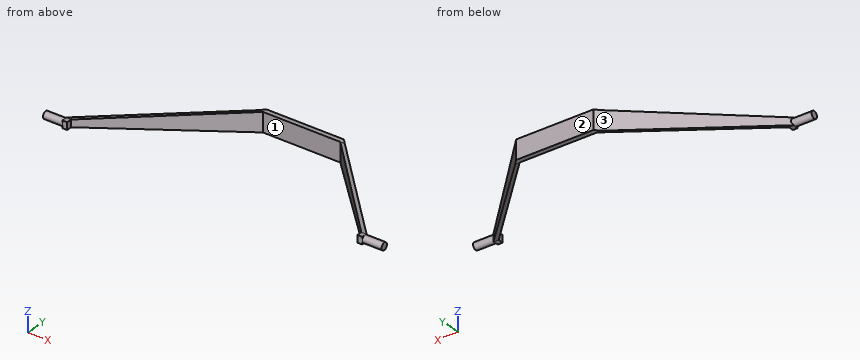
from build123d import *

# Parameters (mm, degrees)
BOSS_EXTRUDE6_DEPTH            = 53.34
BOSS_EXTRUDE6_DEPTH_BACK       = 101.6
CUT_EXTRUDE8_REACH             = 902.262
CUT_EXTRUDE8_DIRECTION_2_REACH = 902.262
SKETCH15_R                     = 19.05
BOSS_EXTRUDE8_DEPTH            = 127
CUT_EXTRUDE9_REACH             = 1709.816
SKETCH16_W                     = 38.1
SKETCH16_H                     = 10.414
CUT_EXTRUDE9_DIRECTION_2_REACH = 1709.816


with BuildPart() as part:
    # Sketch12 → Boss-Extrude6 (new, two sides: drawn at the far end of the back side and taken through both)
    with BuildSketch(Plane.XY.offset(-BOSS_EXTRUDE6_DEPTH_BACK)):
        Polygon((-203.2, 241.3), (203.2, 241.3), (787.471663752, -383.669201703), (787.471663752, -424.309201703), (762.071663752, -424.309201703), (762.071663752, -386.209201703), (203.2, 215.9), (-203.2, 215.9), (-762.071663752, -386.209201703), (-762.071663752, -424.309201703), (-787.471663752, -424.309201703), (-787.471663752, -383.669201703), align=None)
    extrude(amount=BOSS_EXTRUDE6_DEPTH + BOSS_EXTRUDE6_DEPTH_BACK)

    # Cut-Extrude8: up to this plane
    cut_extrude8_end = Plane(origin=(-203.2, 241.3, -101.6), z_dir=(-0.7304911811601322, 0.6829221289775833, 0))
    # Sketch14 → Cut-Extrude8 (cut, up to the surface)
    with BuildSketch(Plane(origin=(0, 0, 0), x_dir=(0, 0, -1), z_dir=(1, 0, 0)), mode=Mode.PRIVATE) as cut_extrude8_sk1:
        Polygon((0, 241.3), (0, 215.9), (-53.34, -386.209201703), (-53.34, 241.3), align=None)
    cut_extrude8_tool1 = split(extrude(cut_extrude8_sk1.sketch, amount=-CUT_EXTRUDE8_REACH, mode=Mode.PRIVATE), bisect_by=cut_extrude8_end, keep=Keep.BOTH, mode=Mode.PRIVATE)
    add(cut_extrude8_tool1.solids().sort_by_distance((0, 31.800889, 34.868308))[0], mode=Mode.SUBTRACT)
    # Sketch14 → Cut-Extrude8 (cut, up to the surface)
    with BuildSketch(Plane(origin=(0, 0, 0), x_dir=(0, 0, -1), z_dir=(1, 0, 0)), mode=Mode.PRIVATE) as cut_extrude8_sk2:
        Polygon((101.6, 215.9), (-15.24, -386.209201703), (-15.24, -424.309201703), (101.6, -424.309201703), align=None)
    cut_extrude8_tool2 = split(extrude(cut_extrude8_sk2.sketch, amount=-CUT_EXTRUDE8_REACH, mode=Mode.PRIVATE), bisect_by=cut_extrude8_end, keep=Keep.BOTH, mode=Mode.PRIVATE)
    add(cut_extrude8_tool2.solids().sort_by_distance((0, -210.192787, -60.465735))[0], mode=Mode.SUBTRACT)

    # Cut-Extrude8 direction 2: up to this plane
    cut_extrude8_direction_2_end = Plane(origin=(203.2, 241.3, -101.6), z_dir=(0.7304911811601321, 0.6829221289775835, 0))
    # Sketch14 → Cut-Extrude8 direction 2 (cut, up to the surface)
    with BuildSketch(Plane(origin=(0, 0, 0), x_dir=(0, 0, -1), z_dir=(1, 0, 0)), mode=Mode.PRIVATE) as cut_extrude8_direction_2_sk1:
        Polygon((0, 241.3), (0, 215.9), (-53.34, -386.209201703), (-53.34, 241.3), align=None)
    cut_extrude8_direction_2_tool1 = split(extrude(cut_extrude8_direction_2_sk1.sketch, amount=CUT_EXTRUDE8_DIRECTION_2_REACH, mode=Mode.PRIVATE), bisect_by=cut_extrude8_direction_2_end, keep=Keep.BOTH, mode=Mode.PRIVATE)
    add(cut_extrude8_direction_2_tool1.solids().sort_by_distance((0, 31.800889, 34.868308))[0], mode=Mode.SUBTRACT)
    # Sketch14 → Cut-Extrude8 direction 2 (cut, up to the surface)
    with BuildSketch(Plane(origin=(0, 0, 0), x_dir=(0, 0, -1), z_dir=(1, 0, 0)), mode=Mode.PRIVATE) as cut_extrude8_direction_2_sk2:
        Polygon((101.6, 215.9), (-15.24, -386.209201703), (-15.24, -424.309201703), (101.6, -424.309201703), align=None)
    cut_extrude8_direction_2_tool2 = split(extrude(cut_extrude8_direction_2_sk2.sketch, amount=CUT_EXTRUDE8_DIRECTION_2_REACH, mode=Mode.PRIVATE), bisect_by=cut_extrude8_direction_2_end, keep=Keep.BOTH, mode=Mode.PRIVATE)
    add(cut_extrude8_direction_2_tool2.solids().sort_by_distance((0, -210.192787, -60.465735))[0], mode=Mode.SUBTRACT)

    # Sketch15 → Boss-Extrude8 (add)
    with BuildSketch(Plane.ZY.offset(762.071663752)):
        with Locations((34.29, -394.845201703)):
            Circle(SKETCH15_R)
    boss_extrude8 = extrude(amount=BOSS_EXTRUDE8_DEPTH)

    # Mirror2: Boss-Extrude8 across plane
    add(boss_extrude8.mirror(Plane(origin=(0, 0, 0), x_dir=(0, 0, 1), z_dir=(1, 0, 0))))

    # Cut-Extrude9: up to this face of the body (flat: up to its plane)
    cut_extrude9_end = Plane(part.part.faces().sort_by_distance((-787.471663752, -416.434815963, 34.29))[0])
    # Sketch16 → Cut-Extrude9 (cut, up to the picked face)
    with BuildSketch(Plane.ZY.offset(762.071663752), mode=Mode.PRIVATE) as cut_extrude9_sk1:
        with Locations((34.29, -419.102201703)):
            Rectangle(SKETCH16_W, SKETCH16_H)
    cut_extrude9_tool1 = split(extrude(cut_extrude9_sk1.sketch, amount=CUT_EXTRUDE9_REACH, mode=Mode.PRIVATE), bisect_by=cut_extrude9_end, keep=Keep.BOTH, mode=Mode.PRIVATE)
    add(cut_extrude9_tool1.solids().sort_by(Axis((-762.071664, -419.102202, 34.29), (-1, 0, 0)))[0], mode=Mode.SUBTRACT)

    # Cut-Extrude9 direction 2: up to this face of the body (flat: up to its plane)
    cut_extrude9_direction_2_end = Plane(part.part.faces().sort_by_distance((787.471663752, -416.434815963, 34.29))[0])
    # Sketch16 → Cut-Extrude9 direction 2 (cut, up to the picked face)
    with BuildSketch(Plane.ZY.offset(762.071663752), mode=Mode.PRIVATE) as cut_extrude9_direction_2_sk1:
        with Locations((34.29, -419.102201703)):
            Rectangle(SKETCH16_W, SKETCH16_H)
    cut_extrude9_direction_2_tool1 = split(extrude(cut_extrude9_direction_2_sk1.sketch, amount=-CUT_EXTRUDE9_DIRECTION_2_REACH, mode=Mode.PRIVATE), bisect_by=cut_extrude9_direction_2_end, keep=Keep.BOTH, mode=Mode.PRIVATE)
    add(cut_extrude9_direction_2_tool1.solids().sort_by(Axis((-762.071664, -419.102202, 34.29), (1, 0, 0)))[0], mode=Mode.SUBTRACT)


solid = part.part
For this review, take the finished solid that the model builds, in its own axes (mm). Face numbers are marked on the shaded views. Round coordinates to 2 decimals unless told otherwise and drop trailing zeros. Order: outer loops, then holes, each group sorted by start corner. A loop starts at its lowest first (then second) coordinate and runs counter-clockwise, first axis right, second up. Notation, with made-up numbers: M 40,-29 L 87,-29 A19 ccw 87,-17 Z; hole C 81.25,-12.5 d9. An arc over 180 degrees is marked long. Use a Markdown table: item, result. Add a question column.
Item 1: Add section B-B, the plane z = -17.5. Give the boundary of the cut face in (x, y).
Item 2: Add section A-A, the plane y = 63. Give the boundary of the cut face in (x, z), then the cut area to 3 significant figures.
Item 3: Insertion check: pin 1 (1 mm diameter, centred on x = 590.5, y = -186, fed in from -Z); pin 2 (2 mm diameter, centred on x = -277, z = -60, fed in from +Y); pin 3 (2 mm diameter, centred on x = -192, z = -73.5, fed in from -Y). Each pin has a flat end and moves straight along its axis. Give the tip position at first contact, or say it passes through.
Item 4: To check wall thickness, follow line 1 along Y through (x, z) = (135.5, -52.5); line 2 along X through (y, z) = (-351.5, 40); line 3 along X through (y, z) = (-114, 21). State the ranges of each line that lie inside material, in increasing order.
Item 5: Mouldability with a two-part tool opening along X and no side actions: class the marked faces 1, 2 and 3 as released by +X, released by -X, zero draft, split by the parting line, or undercut.
Item 6: Add section D-D, the plane x = 572. Give the boundary of the cut face in (y, z).
Item 7: Add section C-C, the plane y = -29.5. Give the boundary of the cut face in (x, z).
Geometry results:
| question | item | result |
|---|---|---|
| 1 | outline | M -632.11,-217.49 L -605.47,-217.49 L -203.2,215.9 L 203.2,215.9 L 605.47,-217.49 L 632.11,-217.49 L 203.2,241.3 L -203.2,241.3 Z |
| 2 | outline | M -369.89,-71.93 L -345.12,-71.93 L -345.12,13.55 L -369.89,13.55 Z; M 345.12,-71.93 L 369.89,-71.93 L 369.89,13.55 L 345.12,13.55 Z |
| 2 | area | 4,230 mm² |
| 3 | pin 1 | stops at z = -23.71 |
| 3 | pin 2 | stops at y = 163.43 |
| 3 | pin 3 | stops at y = 215.9 |
| 4 | line 1 | y = 215.9 to 241.3 |
| 4 | line 2 | x = -757.4 to -729.85, 729.85 to 757.4 |
| 4 | line 3 | x = -535.36 to -509.41, 509.41 to 535.36 |
| 5 | face 1 | undercut |
| 5 | face 2 | zero draft |
| 5 | face 3 | released by -X |
| 6 | outline | M -181.43,-24.5 L -153.19,-29.98 L -153.19,32.7 L -181.43,35.2 Z |
| 7 | outline | M -456.37,-53.98 L -430.98,-53.98 L -430.98,21.74 L -456.37,21.74 Z; M 430.98,-53.98 L 456.37,-53.98 L 456.37,21.74 L 430.98,21.74 Z |
